from build123d import *

# Parameters (mm, degrees)
SKETCH1_W           = 80
SKETCH1_H           = 40
BOSS_EXTRUDE1_DEPTH = 5
SKETCH2_W           = 5
SKETCH2_H           = 40
BOSS_EXTRUDE2_DEPTH = 10
SKETCH3_R           = 2.2
CUT_EXTRUDE1_DEPTH  = 62.881257259
CUT_EXTRUDE2_DEPTH  = 3
BOSS_EXTRUDE3_DEPTH = 40


with BuildPart() as part:
    # Sketch1 → Boss-Extrude1 (new body)
    with BuildSketch(Plane(origin=(0, 0, 0), x_dir=(1, 0, 0), z_dir=(0, 1, 0))):
        Rectangle(SKETCH1_W, SKETCH1_H)
    extrude(amount=BOSS_EXTRUDE1_DEPTH)

    # Sketch2 → Boss-Extrude2 (add)
    with BuildSketch(Plane.XZ):
        with Locations((15.2, 0)):
            Rectangle(SKETCH2_W, SKETCH2_H)
        with Locations((-15.2, 0)):
            Rectangle(SKETCH2_W, SKETCH2_H)
    extrude(amount=BOSS_EXTRUDE2_DEPTH)

    # Sketch3 → Cut-Extrude1 (cut, through all)
    with BuildSketch(Plane.ZY.offset(17.7)):
        with Locations((-10, -5)):
            Circle(SKETCH3_R)
        with Locations((10, -5)):
            Circle(SKETCH3_R)
    extrude(amount=-CUT_EXTRUDE1_DEPTH, mode=Mode.SUBTRACT)

    # Sketch4 → Cut-Extrude2 (cut)
    with BuildSketch(Plane.ZY.offset(17.7)):
        Polygon((-7.892671517, -1.35), (-12.107328483, -1.35), (-14.214656965, -5), (-12.107328483, -8.65), (-7.892671517, -8.65), (-5.785343035, -5), align=None)
        Polygon((12.107328483, -1.35), (7.892671517, -1.35), (5.785343035, -5), (7.892671517, -8.65), (12.107328483, -8.65), (14.214656965, -5), align=None)
    extrude(amount=-CUT_EXTRUDE2_DEPTH, mode=Mode.SUBTRACT)

    # Sketch7 → Boss-Extrude3 (add)
    with BuildSketch(Plane(origin=(0, 0, -20), x_dir=(-1, 0, 0), z_dir=(0, 0, -1))):
        Polygon((0, 70), (0, 60), (12.614253455, 60), (29.537330378, 5), (40, 5), (20, 70), align=None)
        Polygon((-12.614253455, 60), (0, 60), (0, 70), (-20, 70), (-40, 5), (-29.537330378, 5), align=None)
    extrude(amount=-BOSS_EXTRUDE3_DEPTH)

    # Sketch6 → CBORE for 1/4 Square Head Bolt1 (revolve, cut)
    with BuildSketch(Plane(origin=(0, 60, 0), x_dir=(0, 0, -1), z_dir=(1, 0, 0))):
        Polygon((0, 0), (0, 10), (3.3782, 10), (3.3782, 4.7752), (8.33374, 4.7752), (8.33374, 0.635), (8.96874, 0), align=None)
    revolve(axis=Axis((0, 53.65, 0), (0, 1, 0)), mode=Mode.SUBTRACT)


solid = part.part
The listing builds one solid part. Answer for the finished solid, in the listing's coordinates (mm). A direction names the side the tool comes from. Coordinates: 2 decimals unless noted, no trailing zeros. Write each loop counter-clockwise with the first axis right and the second up, starting at its lowest first coordinate (ties: lowest second). Pieces come first, ordered by that corner, then holes. Notation, with made-up numbers: M 34.25,-18 L 90.25,-18 A11 cw 90.25,-14 Z; hole C 19,64.5 d7. An arc over 180 degrees is marked long. Put each result on its own line as item: value. Start each with the question number.
1. A cutting plane is placed at D-D on x = 27. Write down the section's boundary in (y, z), then the cut area to 3 significant figures.
2. Which of the six approach directions +Z, -Z, +X, -X, +Y, -Y give full straight-line access (tool end or side, diameter ignored) to faces 4 (the flat face through (17.7, -5, 0)), 5 (the flat face through (-17.7, -5, 0)), 6 (the cylindrical face through (15.165, -4.903, 7.802)), 7 (the flat face through (0, 0, 0)), 8 (the flat face through (-16, -8.65, 10))?
3. A cutting plane is placed at A-A on x = 0. Write down the section's boundary in (y, z) (3 decimals).
4. Flat-ended cylindrical pins translate along their axes: P1, Ø3, axis at y = 41.5, z = 9.5, coming from the -X side; P2, Ø3, axis at y = -6, z = -1, coming from the +X side; P3, Ø5.5, axis at y = -5, z = 10, coming from the -X side. Find the tip coordinate at first contact, or state that the pin passes through.
5. Consider line 1 (Z direction, x = 0, y = 63); line 2 (Y direction, x = 5, z = -6); line 3 (Y direction, x = 8, z = 12). Determine where each line is inside the solid, lowest interval first. Write a range as from..to.
6. A cutting plane is placed at B-B on z = -10. Count the separate pieces of the cut face and the enclosed holes in it, then the cut area to 3 significant figures.
7. For a pull along Z with two mould halves and no side action, classify faces 1 (the flat face through (0, 5, 0)), 2 (the flat face through (-16.221, -3.201, -6.824)), 3 (the cylindrical face through (15.16, -4.34, -7.9)) as pulls with the +Z half, pulls with the -Z half, needs draft (parallel to the pull), parting line crosses it, or undercut.
8. A cutting plane is placed at C-C on y = 38. Write down the section's boundary in (x, z), then the cut area to 3 significant figures.
Resolved:
1. outline: M 0,-20 L 5,-20 L 5,20 L 0,20 Z; M 13.25,-20 L 47.25,-20 L 47.25,20 L 13.25,20 Z
1. area: 1,560 mm2
2. face 4: +Z, -Z, +X, -Y
2. face 5: +Z, -Z, -X, -Y
2. face 6: +X, -X
2. face 7: +Z, -Z, -Y
2. face 8: -X
3. outline: M 0,-20 L 5,-20 L 5,20 L 0,20 Z; M 60,-20 L 70,-20 L 70,-3.378 L 64.775,-3.378 L 64.775,-8.334 L 60.635,-8.334 L 60,-8.969 Z; M 60,8.969 L 60.635,8.334 L 64.775,8.334 L 64.775,3.378 L 70,3.378 L 70,20 L 60,20 Z
4. P1: stops at x = -29.23
4. P2: stops at x = 17.7
4. P3: stops at x = -14.7
5. line 1: z = -20..-8.33, 8.33..20
5. line 2: y = 0..5, 64.78..70
5. line 3: y = 0..5, 60..70
6. separate pieces: 3
6. enclosed holes: 1
6. area: 2,030 mm2
7. face 1: needs draft
7. face 2: undercut
7. face 3: undercut
8. outline: M -29.85,-20 L -19.38,-20 L -19.38,20 L -29.85,20 Z; M 19.38,-20 L 29.85,-20 L 29.85,20 L 19.38,20 Z
8. area: 837 mm2
